CAD build for the part. Positions are in the model's coordinates, mm. A direction names the side the tool comes from. Round coordinates to 2 decimals unless told otherwise and drop trailing zeros. Order: outer loops, then holes, each group sorted by start corner. A loop starts at its lowest first (then second) coordinate and runs counter-clockwise, first axis right, second up. Notation, with made-up numbers: M -17.5,20 L 28.5,20 A30 cw 28.5,51 Z; hole C 17,9.5 d8. An arc over 180 degrees is marked long. Answer as a JSON object with one key per item and string values.
```python
from build123d import *

# Parameters (mm, degrees)
SKETCH_1_W          = 10
SKETCH_1_H          = 3
EXTRUDE_1_DEPTH     = 3
SKETCH_2_W          = 20
SKETCH_2_H          = 20
CUT_EXTRUDE_1_DEPTH = 10
FILLET_1_R          = 3


with BuildPart() as part:
    # 草图1 → 凸台-拉伸1 (new body)
    with BuildSketch(Plane.XY):
        Polygon((-40, 24), (-35, 24), (-35, 27), (-25, 27), (-25, 24), (-20, 24), (-20, 27), (-10, 27), (-10, 24), (-5, 24), (-5, 27), (5, 27), (5, 24), (10, 24), (10, 27), (20, 27), (20, 24), (25, 24), (25, 27), (35, 27), (35, 24), (40, 24), (40, 21), (43, 21), (43, 11), (40, 11), (40, 6), (43, 6), (43, -4), (40, -4), (40, -9), (43, -9), (43, -19), (40, -19), (40, -24), (-40, -24), (-40, -19), (-43, -19), (-43, -9), (-40, -9), (-40, -4), (-43, -4), (-43, 6), (-40, 6), (-40, 11), (-43, 11), (-43, 21), (-40, 21), align=None)
        with Locations((-15, -20.5)):
            Rectangle(SKETCH_1_W, SKETCH_1_H, mode=Mode.SUBTRACT)
        with Locations((-30, -20.5)):
            Rectangle(SKETCH_1_W, SKETCH_1_H, mode=Mode.SUBTRACT)
        with Locations((0, -20.5)):
            Rectangle(SKETCH_1_W, SKETCH_1_H, mode=Mode.SUBTRACT)
        with Locations((15, -20.5)):
            Rectangle(SKETCH_1_W, SKETCH_1_H, mode=Mode.SUBTRACT)
        with Locations((30, -20.5)):
            Rectangle(SKETCH_1_W, SKETCH_1_H, mode=Mode.SUBTRACT)
    extrude(amount=EXTRUDE_1_DEPTH)

    # 草图2 → 切除-拉伸1 (cut)
    with BuildSketch(Plane.XY.offset(3)):
        Rectangle(SKETCH_2_W, SKETCH_2_H)
    extrude(amount=-CUT_EXTRUDE_1_DEPTH, mode=Mode.SUBTRACT)

    # 圆角1
    fillet_1_edges = [part.edges().sort_by_distance(p)[0] for p in [
        (10, 10, 1.5),
        (10, -10, 1.5),
        (-10, -10, 1.5),
        (-10, 10, 1.5),
    ]]
    fillet(fillet_1_edges, radius=FILLET_1_R)


solid = part.part
```
Item 1: Saw through at A-A on x = -13.5. List the corners of the cut face in (y, z), and give its area (3 significant figures).
Worked answers:
{"outline": "M -24,0 L -22,0 L -22,3 L -24,3 Z; M -19,0 L 27,0 L 27,3 L -19,3 Z", "area": "144 mm2"}
Item 2: Saw through at C-C on z = 1.6. State how many separate pieces and enclosed holes the cut face has, and give its area (3 significant figures).
Worked answers:
{"separate pieces": "1", "enclosed holes": "6", "area": "3,630 mm2"}
Item 3: Saw through at B-B on y = -1. List the corners of the cut face in (x, z), and give its area (3 significant figures).
Worked answers:
{"outline": "M -43,0 L -10,0 L -10,3 L -43,3 Z; M 10,0 L 43,0 L 43,3 L 10,3 Z", "area": "198 mm2"}
Item 4: Saw through at D-D on x = -23. List the corners of the cut face in (y, z), and give its area (3 significant figures).
Worked answers:
{"outline": "M -24,0 L 24,0 L 24,3 L -24,3 Z", "area": "144 mm2"}
Item 5: Drop flat-ended pins along their axis: pin 1 Ø0.9 at (x, z) = (41.5, 2) entering from -Y; pin 2 Ø0.9 at (y, z) = (-20.5, 2) entering from +X; pin 3 Ø1 at (y, z) = (-8, 2.5) entering from -X. Give the stop position or say it passes through.
Worked answers:
{"pin 1": "stops at y = -19", "pin 2": "stops at x = 40", "pin 3": "stops at x = -40"}
Item 6: Two-plate mould, pull along Y, no slides. Class faces 6 (the flat face through (37, 24, 1)), 7 (the flat face through (41, -9, 1)), 8 (the flat face through (-40, 22, 1)): released by +Y, released by -Y, zero draft, split by the parting line, or undercut.
Worked answers:
{"face 6": "released by +Y", "face 7": "undercut", "face 8": "zero draft"}
Item 7: Wall check: line 1 along Y through (x, z) = (-3, 2.4); line 2 along X through (y, z) = (25.5, 1.05); line 3 along Y through (x, z) = (-26.5, 1.35). Give the ranges that are in metal, low to high. Write a range as [from, to].
Worked answers:
{"line 1": "y = [-24, -22], [-19, -10], [10, 27]", "line 2": "x = [-35, -25], [-20, -10], [-5, 5], [10, 20], [25, 35]", "line 3": "y = [-24, -22], [-19, 27]"}
Item 8: 3-axis set-ups, long thin cutter, end or side, ignore diameter. For faces 1 (the flat face through (-41, 11, 1)), 2 (the flat face through (-25, 26, 1)), 3 (the flat face through (-38, 24, 1)), 4 (the flat face through (-41, -19, 1)), 5 (the flat face through (15, -19, 1)): which of +Z, -Z, +X, -X, +Y, -Y reach the whole face in a straight line?
Worked answers:
{"face 1": "+Z, -Z, -X", "face 2": "+Z, -Z, +Y", "face 3": "+Z, -Z, -X, +Y", "face 4": "+Z, -Z, -X, -Y", "face 5": "+Z, -Z"}
